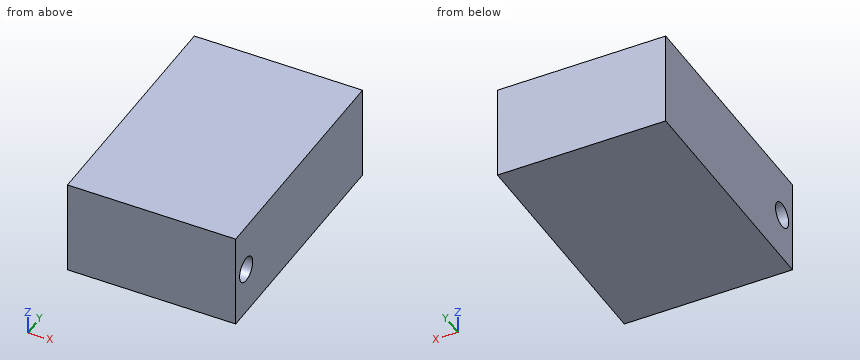
from build123d import *

# Parameters (mm, degrees)
SKETCH2_W               = 85.598
SKETCH2_H               = 123.19
BOSS_EXTRUDE1_DEPTH     = 48.514
CUT_EXTRUDE1_DEPTH      = 158.659131991
CUT_EXTRUDE1_DEPTH_BACK = 158.659131991
SKETCH3_R               = 6.35


with BuildPart() as part:
    # Sketch2 → Boss-Extrude1 (new body)
    with BuildSketch(Plane.XY):
        with Locations((42.799, 61.595)):
            Rectangle(SKETCH2_W, SKETCH2_H)
    extrude(amount=BOSS_EXTRUDE1_DEPTH)

    # Sketch3 → Cut-Extrude1 (cut, two sides: drawn at the far end of the back side and taken through both)
    with BuildSketch(Plane.ZY.offset(-CUT_EXTRUDE1_DEPTH_BACK)):
        with Locations((24.257, 10.16)):
            Circle(SKETCH3_R)
    extrude(amount=CUT_EXTRUDE1_DEPTH + CUT_EXTRUDE1_DEPTH_BACK, mode=Mode.SUBTRACT)


solid = part.part
CAD build for the part. Positions are in the model's coordinates, mm. Round coordinates to 2 decimals unless told otherwise and drop trailing zeros. Order: outer loops, then holes, each group sorted by start corner. A loop starts at its lowest first (then second) coordinate and runs counter-clockwise, first axis right, second up. Notation, with made-up numbers: M 38.5,68 L 93.5,68 A30 ccw 93.5,94 Z; hole C -31.75,89.25 d10. An arc over 180 degrees is marked long. Use one line per item in the form item = value.
Q1. Probe L1, parallel to Z at x = 61, y = 10; L2, parallel to Y at x = 58, z = 20; L3, parallel to Y at x = 5.5, z = 19. List the from-to ranges inside material, lowest first.
Recorded:
L1 = 0 to 17.91, 30.6 to 48.51
L2 = 0 to 5.45, 14.87 to 123.19
L3 = 0 to 6.6, 13.72 to 123.19
Q2. Saw through at B-B on x = 77.5. Give the cut face in (y, z).
Recorded:
outline = M 0,0 L 123.19,0 L 123.19,48.51 L 0,48.51 Z; hole C 10.16,24.26 d12.7
Q3. Saw through at A-A on y = 10.16. Give the cut face in (x, z), then the cut area to 3 significant figures.
Recorded:
outline = M 0,0 L 85.6,0 L 85.6,17.91 L 0,17.91 Z; M 0,30.61 L 85.6,30.61 L 85.6,48.51 L 0,48.51 Z
area = 3,070 mm^2
Q4. Flat gauge pin, fed straight in: P1, Ø11.5, axis at y = 10.16, z = 24.257, coming from the +X side. Where does the tip first touch, or does it go through?
Recorded:
P1 = through
